```python
from build123d import *


with BuildPart() as f2:
    # F2: sweep along a path in F0
    with BuildLine(Plane.XY) as f2_path:
        Line((228.6, -457.2), (228.6, 457.2))
        Line((228.6, 457.2), (-228.6, 457.2))
        Line((-228.6, 457.2), (-228.6, -457.2))
        Line((-228.6, -457.2), (228.6, -457.2))
    # F1 (on Front) → F2 (sweep)
    with BuildSketch(Plane.XZ):
        Polygon((231.775, -3.175), (231.775, 9.525), (228.6, 9.525), (228.6, 0), (219.075, 0), (219.075, -3.175), align=None)
    sweep(path=f2_path.line, transition=Transition.RIGHT)


solid = f2.part
```
Here's how the part is built. I have some questions about the finished solid (model axes, mm). Round coordinates to 2 decimals unless told otherwise and drop trailing zeros. Order: outer loops, then holes, each group sorted by start corner. A loop starts at its lowest first (then second) coordinate and runs counter-clockwise, first axis right, second up. Notation, with made-up numbers: M 48.5,34 L 103.5,34 A18 ccw 103.5,43 Z; hole C 42,-10.5 d1. An arc over 180 degrees is marked long. Use CSV: the item, a comma, the result in double quotes.
1) I want a section at B-B (x = 110.5). List the corners of the cut face in (y, z) for me (3 decimals).
Taken from the geometry:
outline,"M -460.375,-3.175 L -447.675,-3.175 L -447.675,0 L -457.2,0 L -457.2,9.525 L -460.375,9.525 Z; M 447.675,-3.175 L 460.375,-3.175 L 460.375,9.525 L 457.2,9.525 L 457.2,0 L 447.675,0 Z"
2) I want a section at C-C (z = 3). List the corners of the cut face in (x, y) for me (3 decimals).
Taken from the geometry:
outline,"M -231.775,-460.375 L 231.775,-460.375 L 231.775,460.375 L -231.775,460.375 Z; hole M -228.6,-457.2 L 228.6,-457.2 L 228.6,457.2 L -228.6,457.2 Z"
3) If we mould it in two halves opening along X, with no side actions, what happens to faces 1 (the flat face through (222, 2, -3.175)), 2 (the flat face through (221, 2, 0))? For each: pulls with the +X half, pulls with the -X half, needs draft (parallel to the pull), parting line crosses it, or undercut.
Taken from the geometry:
face 1,"needs draft"
face 2,"undercut"
4) I want a section at A-A (y = 111). List the corners of the cut face in (x, z) for me (3 decimals), then the cut area to 3 significant figures.
Taken from the geometry:
outline,"M -231.775,-3.175 L -219.075,-3.175 L -219.075,0 L -228.6,0 L -228.6,9.525 L -231.775,9.525 Z; M 219.075,-3.175 L 231.775,-3.175 L 231.775,9.525 L 228.6,9.525 L 228.6,0 L 219.075,0 Z"
area,"141 mm^2"
5) I need wall thicknesses on line 1 along X through (y, z) = (-243.5, 5.75) (3 decimals); line 2 along Y through (x, z) = (31.5, -1.5) (3 decimals); line 3 along Y through (x, z) = (-40, 0.25) (3 decimals). Which ranges of each line are inside material? Lowest first, please. Write a range as [from, to].
Taken from the geometry:
line 1,"[-231.775, -228.6], [228.6, 231.775]"
line 2,"[-460.375, -447.675], [447.675, 460.375]"
line 3,"[-460.375, -457.2], [457.2, 460.375]"
